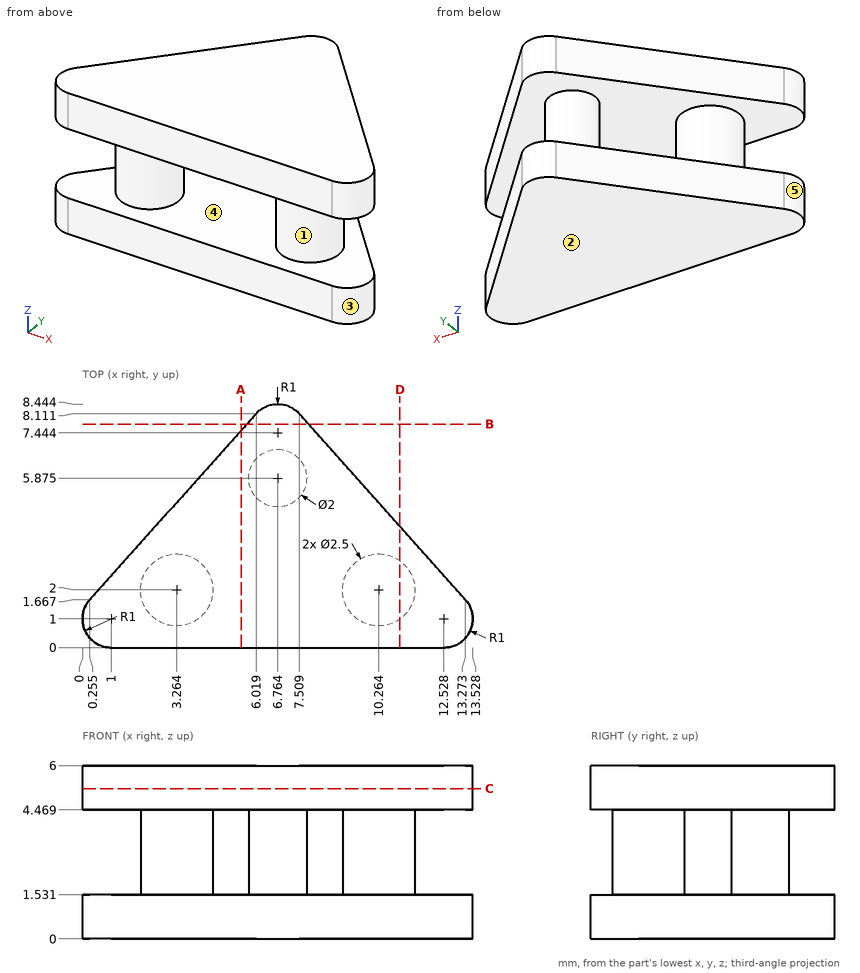
Print and shaded views of the part. All mm, measured from the part's lowest x, y and z. A direction names the side the tool comes from. Coordinates: 2 decimals unless noted, no trailing zeros. Loops run counter-clockwise (first coordinate to the right, second up) from the corner with the lowest first, then second, coordinate; pieces in that order, holes last. Notation, with made-up numbers: (37.25, -8) -> (44.25, -8) arc R25 cw to (44.25, 28) -> close; hole circle Ø8 at (51.5, 13.5). An arc over 180 degrees is marked (long way). Use a Markdown table: item, result. Add a question column.
Item 1: Pull direction Z, two halves, no side cores. Call the marked faces 1, 2 and 3: +Z half, -Z half, draft (parallel to the pull), parting line (faces both ways), or undercut.
Item 2: Band-saw the part on D-D on x = 11. Write the cut outline in (y, z).
Item 3: Band-saw the part on B-B on y = 7.75. Write the cut outline in (x, z) (1 decimal).
Item 4: Band-saw the part on A-A on x = 5.5. Write the cut outline in (y, z).
Item 5: Probe probe 1 along Z at (x, y) = (12.25, 2.5); probe 2 along X at (y, z) = (2.5, 1.35); probe 3 along X at (y, z) = (1, 3.2) (1 decimal). List the from-to ranges inside material, lowest first.
Item 6: Band-saw the part on C-C on z = 5.2. Write the cut outline in (x, y) (1 decimal), plus the area to 3 significant figures.
Item 7: Which spindle directions (+Z, -Z, +X, -X, +Y, -Y) get a long thin tool onto all of the face, cutting with end or side? Do the marked faces 4 and 5. Say none if no direction does.
Geometry says:
| question | item | result |
|---|---|---|
| 1 | face 1 | undercut |
| 1 | face 2 | -Z half |
| 1 | face 3 | draft |
| 2 | outline | (0, 0) -> (4.21, 0) -> (4.21, 1.53) -> (3.01, 1.53) -> (3.01, 4.47) -> (4.21, 4.47) -> (4.21, 6) -> (0, 6) -> (0, 4.47) -> (0.99, 4.47) -> (0.99, 1.53) -> (0, 1.53) -> close |
| 3 | outline | (5.7, 0) -> (7.8, 0) -> (7.8, 1.5) -> (5.7, 1.5) -> close; (5.7, 4.5) -> (7.8, 4.5) -> (7.8, 6) -> (5.7, 6) -> close |
| 4 | outline | (0, 0) -> (7.53, 0) -> (7.53, 1.53) -> (0, 1.53) -> close; (0, 4.47) -> (7.53, 4.47) -> (7.53, 6) -> (0, 6) -> close |
| 5 | probe 1 | 0 to 1.53, 4.47 to 6 |
| 5 | probe 2 | 1 to 12.53 |
| 5 | probe 3 | 2.5 to 4, 9.5 to 11 |
| 6 | outline | (0.3, 1.7) arc R1 ccw to (1, 0) -> (12.5, 0) arc R1 ccw to (13.3, 1.7) -> (7.5, 8.1) arc R1 ccw to (6, 8.1) -> close |
| 6 | area | 69.1 mm² |
| 7 | face 4 | none |
| 7 | face 5 | +Z, -Z, -X |
